```python
from build123d import *

# Parameters (mm, degrees)
SKETCH_W        = 200
SKETCH_H        = 60
PAD_DEPTH       = 2
SKETCH002_R     = 1.6
POCKET001_DEPTH = 5
CHAMFER_SIZE    = 5
SKETCH004_R     = 1.25
POCKET_DEPTH    = 2.001
SKETCH003_W     = 95
SKETCH003_H     = 35
PAD001_DEPTH    = 8
SKETCH005_W     = 42
SKETCH005_H     = 11.5
POCKET002_DEPTH = 10.001
SKETCH006_W     = 70.5
SKETCH006_H     = 20
PAD002_DEPTH    = 14
SKETCH007_R     = 5
SKETCH007_R_2   = 3.75
POCKET003_DEPTH = 16.001


with BuildPart() as part:
    # Sketch → Pad (new body)
    with BuildSketch(Plane.YZ):
        with Locations((100, 30)):
            Rectangle(SKETCH_W, SKETCH_H)
    extrude(amount=PAD_DEPTH)

    # Sketch002 → Pocket001 (cut)
    with BuildSketch(Plane.YZ.offset(2)):
        with Locations((7.5, 52.5)):
            Circle(SKETCH002_R)
        with Locations((7.5, 7.5)):
            Circle(SKETCH002_R)
        with Locations((192.5, 7.5)):
            Circle(SKETCH002_R)
        with Locations((192.5, 52.5)):
            Circle(SKETCH002_R)
    extrude(amount=-POCKET001_DEPTH, mode=Mode.SUBTRACT)

    # Chamfer
    chamfer_edges = [part.edges().sort_by_distance(p)[0] for p in [
        (1, 0, 0),
        (1, 0, 60),
        (1, 200, 60),
        (1, 200, 0),
    ]]
    chamfer(chamfer_edges, length=CHAMFER_SIZE)

    # Sketch004 (on Face5 of Chamfer) → Pocket (cut, through all)
    with BuildSketch(Plane.YZ.offset(2)):
        with Locations((20, 51)):
            Circle(SKETCH004_R)
        with Locations((20, 15)):
            Circle(SKETCH004_R)
        with Locations((181, 15)):
            Circle(SKETCH004_R)
        with Locations((181, 51)):
            Circle(SKETCH004_R)
    extrude(amount=-POCKET_DEPTH, mode=Mode.SUBTRACT)

    # Sketch003 → Pad001 (join)
    with BuildSketch(Plane.YZ.offset(2)):
        with Locations((63, 38)):
            Rectangle(SKETCH003_W, SKETCH003_H)
    extrude(amount=PAD001_DEPTH)

    # Sketch005 (on Face24 of Pad001) → Pocket002 (cut, through all)
    with BuildSketch(Plane.YZ.offset(10)):
        with Locations((40.5, 39.75)):
            Rectangle(SKETCH005_W, SKETCH005_H)
        with Locations((85.5, 39.75)):
            Rectangle(SKETCH005_W, SKETCH005_H)
    extrude(amount=-POCKET002_DEPTH, mode=Mode.SUBTRACT)

    # Sketch006 (on Face5 of Pocket002) → Pad002 (join)
    with BuildSketch(Plane.YZ.offset(2)):
        with Locations((145.75, 41)):
            Rectangle(SKETCH006_W, SKETCH006_H)
    extrude(amount=PAD002_DEPTH)

    # Sketch007 (on Face2 of Pad002) → Pocket003 (cut, through all)
    with BuildSketch(Plane(origin=(0, 0, 0), x_dir=(0, 1, 0), z_dir=(-1, 0, 0))):
        with Locations((169.9, -40.375)):
            Circle(SKETCH007_R)
        with Locations((144.9, -40.375)):
            Circle(SKETCH007_R_2)
        with Locations((122.4, -40.375)):
            Circle(SKETCH007_R_2)
    extrude(amount=-POCKET003_DEPTH, mode=Mode.SUBTRACT)


with BuildPart() as part_1:
    # Body placement: moved
    add(part.part.moved(Location((0, 1.067224, 0))))


solid = part_1.part
```
CAD build for the part. Positions are in the model's coordinates, mm. A direction names the side the tool comes from. Round coordinates to 2 decimals unless told otherwise and drop trailing zeros. Order: outer loops, then holes, each group sorted by start corner. A loop starts at its lowest first (then second) coordinate and runs counter-clockwise, first axis right, second up.
Item 1: Saw through at D-D on x = 12. Write the cut outline in (y, z) (3 decimals), then the cut area to 3 significant figures.
Item 2: Tool access for faces 1 (the face through (5, 41, 34)), 2 (the face through (9, 146, 51)), 3 (the face through (9, 146, 31)), 4 (the face through (13, 111.567, 41)), 5 (the face through (6, 63, 20.5)): list every direction of +Z, -Z, +X, -X, +Y, -Y with a clear straight run to the whole face (end or side of a thin tool).
Item 3: Saw through at B-B on z = 24.5. Write the cut outline in (x, y).
Item 4: Probe line 1 along Z through (x, y) = (9.5, 23); line 2 along Y through (x, z) = (8.5, 23); line 3 along Z through (x, y) = (1.25, 88.5). List the from-to ranges inside material, lowest first.
Item 5: Saw through at C-C on y = 129.5. Write the cut outline in (x, z), then the cut area to 3 significant figures.
Item 6: Mould opens along Y. For faces 6 (the face through (0, 100, 30)), 7 (the face through (6, 111.567, 53)), 8 (the face through (5, 41, 45.5)), 9 (the face through (1.01, 6.97, 52.57)) say: pulls with the +Y half, pulls with the -Y half, needs draft (parallel to the pull), parting line crosses it, or undercut.
Item 7: Saw through at A-A on y = 46. Write the cut outline in (x, z).
Item 8: Pin check, flat tips, straight feed: pin 1 (4 mm diameter, centred on x = 9.5, y = 159, fed in from +Z); pin 2 (3 mm diameter, centred on x = 4.5, y = 91, fed in from +Z); pin 3 (10 mm diameter, centred on y = 42.5, z = 25.5, fed in from +X); pin 4 (4.5 mm diameter, centred on y = 123.47, z = 40.38, fed in from -X). Stop position of each tip, or through.
Reported:
1. outline: (111.567, 31) - (182.067, 31) - (182.067, 51) - (111.567, 51) - close; hole circle Ø7.5 at (123.467, 40.375); hole circle Ø7.5 at (145.967, 40.375); hole circle Ø10 at (170.967, 40.375)
1. area: 1,240 mm2
2. face 1: +X, -X
2. face 2: +Z, +X, +Y
2. face 3: -Z, +X, +Y
2. face 4: +Z, -Z, +X, -Y
2. face 5: -Z, +X, +Y, -Y
3. outline: (0, 1.07) - (2, 1.07) - (2, 16.57) - (10, 16.57) - (10, 111.57) - (2, 111.57) - (2, 201.07) - (0, 201.07) - close
4. line 1: z = 20.5 to 34, 45.5 to 55.5
4. line 2: y = 16.57 to 111.57
4. line 3: z = 0 to 34, 45.5 to 60
5. outline: (0, 0) - (2, 0) - (2, 31) - (16, 31) - (16, 51) - (2, 51) - (2, 60) - (0, 60) - close
5. area: 400 mm2
6. face 6: needs draft
6. face 7: pulls with the +Y half
6. face 8: undercut
6. face 9: undercut
7. outline: (0, 0) - (2, 0) - (2, 20.5) - (10, 20.5) - (10, 34) - (0, 34) - close; (0, 45.5) - (10, 45.5) - (10, 55.5) - (2, 55.5) - (2, 60) - (0, 60) - close
8. pin 1: stops at z = 51
8. pin 2: stops at z = 55.5
8. pin 3: stops at x = 10
8. pin 4: passes through
